Here's how the part is built. I have some questions about the finished solid (model axes, mm). A direction names the side the tool comes from. Coordinates: 2 decimals unless noted, no trailing zeros. Write each loop counter-clockwise with the first axis right and the second up, starting at its lowest first coordinate (ties: lowest second). Pieces come first, ordered by that corner, then holes.
Item 1: If we section it at C-C (y = 9.25): Please give me the cut outline in (x, z).
Item 2: I'm going to push flat-ended pins straight in: pin 1 Ø2.5 at (y, z) = (9, 34.5) entering from +X; pin 2 Ø2.5 at (x, z) = (40.5, -31.5) entering from +Y; pin 3 Ø6 at (x, z) = (9, 22.5) entering from -Y. Where does each tip first touch, or does it pass through?
Item 3: We'd pull the mould along Z, two halves only. Please class faces 1 (the face through (38.59, 0.99, -34.44)), 2 (the face through (-39, 7, 28.75)), 3 (the face through (-39, 7, -28.75)), 4 (the face through (-43.1, 6, 1)): +Z half, -Z half, draft (parallel to the pull), parting line (faces both ways), or undercut.
Item 4: If we section it at A-A (z = 33.25): Please give me the cut outline in (x, y).
Item 5: If we section it at B-B (x = -39.5): Please give me the cut outline in (y, z).
Item 6: For faces 5 (the face through (-34.6, 7, -33)), 6 (the face through (-34.6, 7, 33)), 7 (the face through (39, 7, 28.75)), which set-ups out of +Z, -Z, +X, -X, +Y, -Y let a thin tool reach every point of the face, with its end or its side?
Item 7: If I drill on line 1 (X direction, y = 1.35, z = -33.25); line 2 (Y direction, x = 38, z = 31.5); line 3 (X direction, y = 4.25, z = 34), over which ranges is the centre line in solid material (lowest first)?
from build123d import *

# Parameters (mm, degrees)
SKETCH_1_W      = 86.2
SKETCH_1_H      = 73.7
SKETCH_1_R      = 1.5
EXTRUDE_1_DEPTH = 2
EXTRUDE_2_DEPTH = 10


with BuildPart() as part:
    # 草图1 → 凸台-拉伸1 (new body)
    with BuildSketch(Plane(origin=(0, 0, 0), x_dir=(1, 0, 0), z_dir=(0, 1, 0))):
        Rectangle(SKETCH_1_W, SKETCH_1_H)
        with Locations(Location((-39.5, 33.25, 0), (0, 0, 270))):
            Circle(SKETCH_1_R, mode=Mode.SUBTRACT)
        with Locations(Location((39.5, 33.25, 0), (0, 0, 270))):
            Circle(SKETCH_1_R, mode=Mode.SUBTRACT)
        with Locations(Location((-39.5, -33.25, 0), (0, 0, 270))):
            Circle(SKETCH_1_R, mode=Mode.SUBTRACT)
        with Locations(Location((39.5, -33.25, 0), (0, 0, 270))):
            Circle(SKETCH_1_R, mode=Mode.SUBTRACT)
    extrude(amount=EXTRUDE_1_DEPTH)

    # 草图2 → 凸台-拉伸2 (add)
    with BuildSketch(Plane(origin=(0, 2, 0), x_dir=(1, 0, 0), z_dir=(0, 1, 0))):
        Polygon((-34.6, 36.85), (34.6, 36.85), (34.6, 28.75), (43.1, 28.75), (43.1, -28.75), (34.6, -28.75), (34.6, -36.85), (-34.6, -36.85), (-34.6, -28.75), (-43.1, -28.75), (-43.1, 28.75), (-34.6, 28.75), align=None)
    extrude(amount=EXTRUDE_2_DEPTH)


solid = part.part
Answer list:
1. outline: (-43.1, -28.75) - (-34.6, -28.75) - (-34.6, -36.85) - (34.6, -36.85) - (34.6, -28.75) - (43.1, -28.75) - (43.1, 28.75) - (34.6, 28.75) - (34.6, 36.85) - (-34.6, 36.85) - (-34.6, 28.75) - (-43.1, 28.75) - close
2. pin 1: stops at x = 34.6
2. pin 2: stops at y = 2
2. pin 3: stops at y = 0
3. face 1: undercut
3. face 2: +Z half
3. face 3: -Z half
3. face 4: draft
4. outline: (-43.1, 0) - (-41, 0) - (-41, 2) - (-43.1, 2) - close; (-38, 0) - (38, 0) - (38, 2) - (34.6, 2) - (34.6, 12) - (-34.6, 12) - (-34.6, 2) - (-38, 2) - close; (41, 0) - (43.1, 0) - (43.1, 2) - (41, 2) - close
5. outline: (0, -36.85) - (2, -36.85) - (2, -34.75) - (0, -34.75) - close; (0, -31.75) - (2, -31.75) - (2, -28.75) - (12, -28.75) - (12, 28.75) - (2, 28.75) - (2, 31.75) - (0, 31.75) - close; (0, 34.75) - (2, 34.75) - (2, 36.85) - (0, 36.85) - close
6. face 5: -Z, -X, +Y
6. face 6: +Z, -X, +Y
6. face 7: +Z, +X, +Y
7. line 1: x = -43.1 to -41, -38 to 38, 41 to 43.1
7. line 2: y = 0 to 2
7. line 3: x = -34.6 to 34.6
